Geometry check sheet. Reference: the model listing, model coordinates, mm. Give positions to 0.01 mm unless a question says otherwise; leave off trailing zeros. Loops run counter-clockwise (first coordinate to the right, second up) from the corner with the lowest first, then second, coordinate; pieces in that order, holes last.
```python
from build123d import *

# Parameters (mm, degrees)
SKETCH1_W           = 57.9
SKETCH1_H           = 76.2
BOSS_EXTRUDE1_DEPTH = 2
SKETCH2_R           = 2
SKETCH2_W           = 12
SKETCH2_H           = 10
SKETCH2_R_2         = 1.5
CUT_EXTRUDE1_DEPTH  = 2
SKETCH4_R           = 2
SKETCH4_R_2         = 1.5
SKETCH4_R_3         = 1.957178151
BOSS_EXTRUDE5_DEPTH = 2
SKETCH8_W           = 57.9
SKETCH8_H           = 76.2
SKETCH8_R           = 2
SKETCH8_R_2         = 1.5
SKETCH8_W_2         = 12
SKETCH8_H_2         = 10
BOSS_EXTRUDE6_DEPTH = 10
SKETCH9_R           = 2
CUT_EXTRUDE6_DEPTH  = 10
SKETCH10_W          = 57.9
SKETCH10_H          = 76.2
CUT_EXTRUDE7_DEPTH  = 10
SKETCH11_W          = 45.093614326
SKETCH11_H          = 27.476395826
BOSS_EXTRUDE7_DEPTH = 2


with BuildPart() as part:
    # Sketch1 → Boss-Extrude1 (new body)
    with BuildSketch(Plane.XY):
        with Locations((-6.590392234, -8.896581688)):
            Rectangle(SKETCH1_W, SKETCH1_H)
    extrude(amount=BOSS_EXTRUDE1_DEPTH)

    # Sketch2 → Cut-Extrude1 (cut)
    with BuildSketch(Plane(origin=(0, 0, 0), x_dir=(-1, 0, 0), z_dir=(0, 0, -1))):
        with Locations((-6.409607766, 14.203418312)):
            Circle(SKETCH2_R)
        with Locations((19.590392234, 14.203418312)):
            Circle(SKETCH2_R)
        with Locations((2.640392234, 4.203418312)):
            Rectangle(SKETCH2_W, SKETCH2_H)
        with Locations((16.590392234, -41.996581688)):
            Circle(SKETCH2_R)
        with Locations((-3.409607766, -41.996581688)):
            Circle(SKETCH2_R)
        with Locations((21.790392234, -13.626581688)):
            Circle(SKETCH2_R_2)
    extrude(amount=-CUT_EXTRUDE1_DEPTH, mode=Mode.SUBTRACT)

    # Sketch4 → Boss-Extrude5 (add)
    # profile 1 of 3: a face of its own
    with BuildSketch(Plane(origin=(0, 0, 0), x_dir=(-1, 0, 0), z_dir=(0, 0, -1))):
        Polygon((35.540392234, 29.203418312), (6.590392234, 29.203418312), (-22.359607766, 29.203418312), (-22.359607766, -46.996581688), (35.540392234, -46.996581688), align=None)
        with Locations((-3.409607766, -41.996581688)):
            Circle(SKETCH4_R, mode=Mode.SUBTRACT)
        with Locations((16.590392234, -41.996581688)):
            Circle(SKETCH4_R, mode=Mode.SUBTRACT)
        with Locations((21.790392234, -13.626581688)):
            Circle(SKETCH4_R_2, mode=Mode.SUBTRACT)
        Polygon((-13.650237399, 24.487372027), (6.590392234, 24.487372027), (30.150370064, 24.487372027), (30.150370064, 9.203418312), (8.640392234, 9.203418312), (8.640392234, -0.796581688), (-3.359607766, -0.796581688), (-3.359607766, 9.203418312), (-13.650237399, 9.203418312), align=None, mode=Mode.SUBTRACT)
    # profile 2 of 3: a face of its own
    with BuildSketch(Plane(origin=(0, 0, 0), x_dir=(-1, 0, 0), z_dir=(0, 0, -1))):
        with Locations((-6.409607766, 14.203418312)):
            Circle(SKETCH4_R)
    # profile 3 of 3: a face of its own
    with BuildSketch(Plane(origin=(0, 0, 0), x_dir=(-1, 0, 0), z_dir=(0, 0, -1))):
        with Locations((19.590392234, 14.203418312)):
            Circle(SKETCH4_R_3)
    extrude(amount=-BOSS_EXTRUDE5_DEPTH)


with BuildPart() as boss_extrude5_piece_1:
    # of the separate pieces the step leaves, piece 1, a body of its own (boss_extrude5_pieces)
    add(part.part.solids().sort_by_distance((-35.540392234, 29.203418312, 0))[0])



with BuildPart() as boss_extrude5_piece_2:
    # of the separate pieces the step leaves, piece 2, a body of its own (boss_extrude5_pieces)
    add(part.part.solids().sort_by_distance((-21.547570385, 14.203418312, 0))[0])


with BuildPart() as boss_extrude5_piece_1_1:
    add(boss_extrude5_piece_1.part)

    add(boss_extrude5_piece_2.part)  # Boss-Extrude6 merges Boss-Extrude5 piece 2
    # Sketch8 → Boss-Extrude6 (add)
    # profile 1 of 2: a face of its own
    with BuildSketch(Plane(origin=(0, 0, 0), x_dir=(-1, 0, 0), z_dir=(0, 0, -1))):
        with Locations((6.590392234, -8.896581688)):
            Rectangle(SKETCH8_W, SKETCH8_H)
        with Locations((16.590392234, -41.996581688)):
            Circle(SKETCH8_R, mode=Mode.SUBTRACT)
        with Locations((21.790392234, -13.626581688)):
            Circle(SKETCH8_R_2, mode=Mode.SUBTRACT)
        with Locations((19.590392234, 14.203418312)):
            Circle(SKETCH8_R, mode=Mode.SUBTRACT)
        with Locations((-3.409607766, -41.996581688)):
            Circle(SKETCH8_R, mode=Mode.SUBTRACT)
        with Locations((2.640392234, 4.203418312)):
            Rectangle(SKETCH8_W_2, SKETCH8_H_2, mode=Mode.SUBTRACT)
    # profile 2 of 2: a face of its own
    with BuildSketch(Plane(origin=(0, 0, 0), x_dir=(-1, 0, 0), z_dir=(0, 0, -1))):
        with Locations((19.590392234, 14.203418312)):
            Circle(SKETCH8_R)
    extrude(amount=BOSS_EXTRUDE6_DEPTH)

    # Sketch9 → Cut-Extrude6 (cut)
    with BuildSketch(Plane(origin=(0, 0, -10), x_dir=(-1, 0, 0), z_dir=(0, 0, -1))):
        with Locations((-6.468155069, 18.203418312)):
            Circle(SKETCH9_R)
        with Locations((19.531844931, 18.203418312)):
            Circle(SKETCH9_R)
    extrude(amount=-CUT_EXTRUDE6_DEPTH, mode=Mode.SUBTRACT)

    # Sketch10 → Cut-Extrude7 (cut)
    with BuildSketch(Plane.XY.offset(2)):
        with Locations((-6.590392234, -8.896581688)):
            Rectangle(SKETCH10_W, SKETCH10_H)
    extrude(amount=-CUT_EXTRUDE7_DEPTH, mode=Mode.SUBTRACT)

    # Sketch11 → Boss-Extrude7 (add)
    with BuildSketch(Plane.XY.offset(-8)):
        with Locations((-7.118685328, 9.132915536)):
            Rectangle(SKETCH11_W, SKETCH11_H)
    extrude(amount=-BOSS_EXTRUDE7_DEPTH)


solid = boss_extrude5_piece_1_1.part
```
1) Mould release check, pull along X, two halves, no side actions. Record for faces 1 (the cylindrical face through (-20.29, -13.56, -8.99)), 2 (the flat face through (-6, -46.997, -9)), 3 (the flat face through (22.36, -9, -9)): +X half, -X half, draft (parallel to the pull), parting line (faces both ways), or undercut.
2) Sectioned sample at A-A on x = -16. Enter the section's corners in (y, z).
3) Scan line: line 1 along Y through (x, z) = (5, -8.9). Record every from-to range of solid material in increasing order.
Determined:
1. face 1: undercut
1. face 2: draft
1. face 3: +X half
2. outline: (-47, -10) - (-43.91, -10) - (-43.91, -8) - (-47, -8) - close; (-40.09, -10) - (29.2, -10) - (29.2, -8) - (-40.09, -8) - close
3. line 1: y = -47 to -43.21, -40.78 to 29.2
